```python
from build123d import *

# Parameters (mm, degrees)
SKETCH_1_W      = 190
SKETCH_1_H      = 490
EXTRUDE_1_DEPTH = 10
EXTRUDE_2_DEPTH = 500
SKETCH_3_W      = 150
SKETCH_3_H      = 160
EXTRUDE_3_DEPTH = 10


with BuildPart() as part:
    # Эскиз1 → Бобышка-Вытянуть1 (new body)
    with BuildSketch(Plane.XY):
        with Locations((95, 245)):
            Rectangle(SKETCH_1_W, SKETCH_1_H)
    extrude(amount=EXTRUDE_1_DEPTH)

    # Эскиз2 → Бобышка-Вытянуть2 (add)
    with BuildSketch(Plane(origin=(0, 0, 0), x_dir=(-1, 0, 0), z_dir=(0, 0, -1))):
        Polygon((-170, 180), (-170, 20), (-20, 20), (-20, 180), (-30, 180), (-30, 30), (-160, 30), (-160, 180), align=None)
    extrude(amount=EXTRUDE_2_DEPTH)

    # Эскиз3 → Бобышка-Вытянуть3 (add)
    with BuildSketch(Plane(origin=(0, 0, -500), x_dir=(-1, 0, 0), z_dir=(0, 0, -1))):
        with Locations((-95, 100)):
            Rectangle(SKETCH_3_W, SKETCH_3_H)
    extrude(amount=EXTRUDE_3_DEPTH)


solid = part.part
```
The listing builds one solid part. Answer for the finished solid, in the listing's coordinates (mm). A direction names the side the tool comes from. Give positions to 0.01 mm unless a question says otherwise; leave off trailing zeros. Loops run counter-clockwise (first coordinate to the right, second up) from the corner with the lowest first, then second, coordinate; pieces in that order, holes last. Notation, with made-up numbers: M 63.25,37.5 L 79.25,37.5 A20 ccw 79.25,42.5 Z; hole C 32,-35.75 d7. An arc over 180 degrees is marked long. One line per item, written item: value.
Q1. Determine the mould class of faces 1 (the face through (96, 101, -510)), 2 (the face through (94, 248, 10)), 3 (the face through (96, 106, -500)) for opening direction Z: +Z half, -Z half, draft (parallel to the pull), parting line (faces both ways), or undercut.
Working result:
face 1: -Z half
face 2: +Z half
face 3: undercut
Q2. A cutting plane is placed at C-C on z = -32. Determine the outline of the cut face in (x, y), then the cut area to 3 significant figures.
Working result:
outline: M 20,20 L 170,20 L 170,180 L 160,180 L 160,30 L 30,30 L 30,180 L 20,180 Z
area: 4,500 mm^2
Q3. A cutting plane is placed at A-A on y = 39. Determine the outline of the cut face in (x, z).
Working result:
outline: M 0,0 L 20,0 L 20,-510 L 170,-510 L 170,0 L 190,0 L 190,10 L 0,10 Z; hole M 30,-500 L 160,-500 L 160,0 L 30,0 Z
Q4. Find the intervals of material crossed by line 1 (X direction, y = 136, z = -378); line 2 (Z direction, x = 97, y = 178); line 3 (Y direction, x = 67, z = -488.5), in increasing order. Write a range as from..to.
Working result:
line 1: x = 20..30, 160..170
line 2: z = -510..-500, 0..10
line 3: y = 20..30
Q5. A cutting plane is placed at D-D on y = 228.5. Determine the outline of the cut face in (x, z), then the cut area to 3 significant figures.
Working result:
outline: M 0,0 L 190,0 L 190,10 L 0,10 Z
area: 1,900 mm^2
Q6. For faces 4 (the face through (170, 99, -251)), 5 (the face through (20, 99, -251)), 6 (the face through (94, 30, -246)), 7 (the face through (162, 180, -254)), 8 (the face through (96, 20, -251)), determine the directions among +Z, -Z, +X, -X, +Y, -Y from which every point of the face is accessible in a straight line to the end or side of a thin tool.
Working result:
face 4: -Z, +X, +Y, -Y
face 5: -Z, -X, +Y, -Y
face 6: +Y
face 7: -Z, +X, -X, +Y
face 8: -Z, +X, -X, -Y
Q7. Flat-ended cylindrical pins translate along their axes: P1, Ø1, axis at x = 100, z = -438.5, coming from the +Y side; P2, Ø12, axis at x = 27, z = -221.5, coming from the -Y side; P3, Ø3, axis at y = 171.5, z = -138, coming from the -X side. Find the tip coordinate at first contact, or state that the pin passes through.
Working result:
P1: stops at y = 30
P2: stops at y = 20
P3: stops at x = 20
Q8. A cutting plane is placed at B-B on x = 49.5. Determine the outline of the cut face in (y, z), then the cut area to 3 significant figures.
Working result:
outline: M 0,0 L 20,0 L 20,-510 L 180,-510 L 180,-500 L 30,-500 L 30,0 L 490,0 L 490,10 L 0,10 Z
area: 11,500 mm^2
